```python
from build123d import *

# Parameters (mm, degrees)
SKETCH1_W          = 148.59
SKETCH1_H          = 102.87
EXTRUDE1_DEPTH     = 32.512
SKETCH2_W          = 6.35
SKETCH2_H          = 102.87
CUT_EXTRUDE1_DEPTH = 25.4
LPATTERN1_COUNT    = 18
LPATTERN1_PITCH    = 8.1788
SKETCH3_R          = 2.286
CUT_EXTRUDE2_DEPTH = 78.74
SKETCH4_W          = 1.8288
SKETCH4_H          = 19.05
CUT_EXTRUDE3_DEPTH = 25.4


with BuildPart() as part:
    # Sketch1 → Extrude1 (new body)
    with BuildSketch(Plane(origin=(0, 0, 0), x_dir=(1, 0, 0), z_dir=(0, 1, 0))):
        with Locations((74.295, 51.435)):
            Rectangle(SKETCH1_W, SKETCH1_H)
    extrude(amount=EXTRUDE1_DEPTH)

    # Sketch2 → Cut-Extrude1 (cut)
    with BuildSketch(Plane(origin=(0, 32.512, 0), x_dir=(-1, 0, 0), z_dir=(0, 1, 0))):
        with Locations((-4.7625, -51.435)):
            Rectangle(SKETCH2_W, SKETCH2_H)
    cut_extrude1 = extrude(amount=-CUT_EXTRUDE1_DEPTH, mode=Mode.SUBTRACT)

    # LPattern1: Cut-Extrude1 ×18
    with Locations(*[(i * LPATTERN1_PITCH, 0, 0) for i in range(1, LPATTERN1_COUNT)]):
        add(cut_extrude1, mode=Mode.SUBTRACT)

    # Sketch3 → Cut-Extrude2 (cut)
    with BuildSketch(Plane.XZ):
        with Locations(Location((33.5788, -6.35, 0), (0, 0, 270))):
            Circle(SKETCH3_R)
        with Locations(Location((33.5788, -94.742, 0), (0, 0, 270))):
            Circle(SKETCH3_R)
        with Locations(Location((116.1288, -6.35, 0), (0, 0, 270))):
            Circle(SKETCH3_R)
        with Locations(Location((116.1288, -94.742, 0), (0, 0, 270))):
            Circle(SKETCH3_R)
    extrude(amount=-CUT_EXTRUDE2_DEPTH, mode=Mode.SUBTRACT)

    # Sketch4 → Cut-Extrude3 (cut)
    with BuildSketch(Plane(origin=(0, 32.512, 0), x_dir=(-1, 0, 0), z_dir=(0, 1, 0))):
        with Locations((-33.3883, -93.345)):
            Rectangle(SKETCH4_W, SKETCH4_H)
        with Locations((-115.1763, -93.345)):
            Rectangle(SKETCH4_W, SKETCH4_H)
        with Locations((-33.3883, -9.525)):
            Rectangle(SKETCH4_W, SKETCH4_H)
        with Locations((-115.1763, -9.525)):
            Rectangle(SKETCH4_W, SKETCH4_H)
    extrude(amount=-CUT_EXTRUDE3_DEPTH, mode=Mode.SUBTRACT)


solid = part.part
```
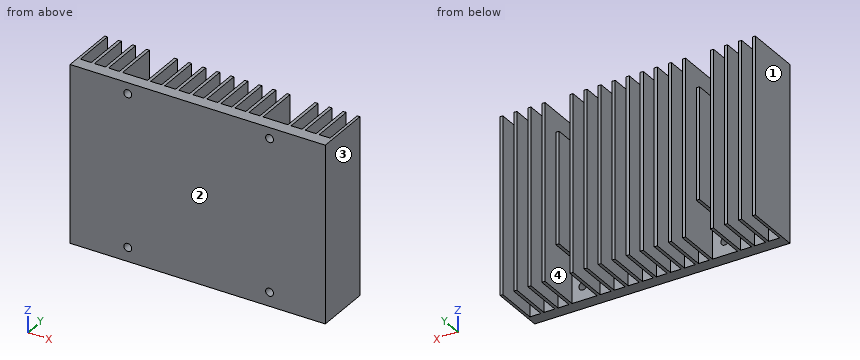
For this review, take the finished solid that the model builds, in its own axes (mm). Face numbers are marked on the shaded views. Coordinates: 2 decimals unless noted, no trailing zeros. Write each loop counter-clockwise with the first axis right and the second up, starting at its lowest first coordinate (ties: lowest second). Pieces come first, ordered by that corner, then holes.
(1) For pin 1 Ø1 at (x, y) = (31.5, 20) entering from -Z; pin 2 Ø7.5 at (x, z) = (116.13, -94.74) entering from +Y, all flat-tipped, find the tip position at first contact; note any pin that passes through.
(2) The part is to be moulded in two halves that separate along X. For the marked faces 1, 2, 3 and 4, say which applies: +X half, -X half, draft (parallel to the pull), parting line (faces both ways), or undercut.
(3) Add section B-B on x = 39. Give the boundary of the cut face in (y, z), then the cut area to 3 significant figures.
(4) Wall thickness on probe 1 along X at (y, z) = (5.75, -6.35); probe 2 along Y at (x, z) = (114, -27); probe 3 along Z at (x, y) = (116, 21): over which ranges is each line inside the solid? List them lowest first.
(5) Add section A-A on z = -6.35. Count the separate pieces of the cut face and the enclosed holes in it, then the cut area to 3 significant figures.
Answer sheet:
1. pin 1: passes through
1. pin 2: stops at y = 7.11
2. face 1: -X half
2. face 2: draft
2. face 3: +X half
2. face 4: undercut
3. outline: (0, -102.87) - (7.11, -102.87) - (7.11, 0) - (0, 0) - close
3. area: 732 mm2
4. probe 1: x = 0 to 31.29, 35.86 to 113.84, 118.41 to 148.59
4. probe 2: y = 0 to 7.11
4. probe 3: z = -83.82 to -19.05
5. separate pieces: 3
5. enclosed holes: 0
5. area: 1,770 mm2
